```python
from build123d import *

# Parameters (mm, degrees)
SKETCH1_R           = 27.5
SKETCH1_R_2         = 2.5
BOSS_EXTRUDE1_DEPTH = 4
SKETCH2_R           = 11
CUT_EXTRUDE1_DEPTH  = 15
BOSS_EXTRUDE3_START = -4
SKETCH3_R           = 2.5
SKETCH3_R_2         = 1.875
BOSS_EXTRUDE3_DEPTH = 4


with BuildPart() as part:
    # Sketch1 → Boss-Extrude1 (new body)
    with BuildSketch(Plane(origin=(0, 0, 0), x_dir=(1, 0, 0), z_dir=(0, 1, 0))):
        with Locations(Location((0, 0, 0), (0, 0, 270))):
            Circle(SKETCH1_R)
        with Locations(Location((0, 20, 0), (0, 0, 270))):
            Circle(SKETCH1_R_2, mode=Mode.SUBTRACT)
        with Locations(Location((-20, 0, 0), (0, 0, 270))):
            Circle(SKETCH1_R_2, mode=Mode.SUBTRACT)
        with Locations(Location((20, 0, 0), (0, 0, 270))):
            Circle(SKETCH1_R_2, mode=Mode.SUBTRACT)
        with Locations(Location((0, -20, 0), (0, 0, 270))):
            Circle(SKETCH1_R_2, mode=Mode.SUBTRACT)
    extrude(amount=BOSS_EXTRUDE1_DEPTH)

    # Sketch2 → Cut-Extrude1 (cut)
    with BuildSketch(Plane(origin=(0, 4, 0), x_dir=(1, 0, 0), z_dir=(0, 1, 0))):
        with Locations(Location((0, 0, 0), (0, 0, 270))):
            Circle(SKETCH2_R)
    extrude(amount=-CUT_EXTRUDE1_DEPTH, mode=Mode.SUBTRACT)

    # Sketch3 → Boss-Extrude3 (add)
    # profile 1 of 4: a face of its own
    with BuildSketch(Plane(origin=(0, 4, 0), x_dir=(1, 0, 0), z_dir=(0, 1, 0)).offset(BOSS_EXTRUDE3_START)):
        with Locations((0, -20)):
            Circle(SKETCH3_R)
        with Locations(Location((0, -20, 0), (0, 0, 270))):
            Circle(SKETCH3_R_2, mode=Mode.SUBTRACT)
    # profile 2 of 4: a face of its own
    with BuildSketch(Plane(origin=(0, 4, 0), x_dir=(1, 0, 0), z_dir=(0, 1, 0)).offset(BOSS_EXTRUDE3_START)):
        with Locations((20, 0)):
            Circle(SKETCH3_R)
        with Locations(Location((20, 0, 0), (0, 0, 270))):
            Circle(SKETCH3_R_2, mode=Mode.SUBTRACT)
    # profile 3 of 4: a face of its own
    with BuildSketch(Plane(origin=(0, 4, 0), x_dir=(1, 0, 0), z_dir=(0, 1, 0)).offset(BOSS_EXTRUDE3_START)):
        with Locations((0, 20)):
            Circle(SKETCH3_R)
        with Locations(Location((0, 20, 0), (0, 0, 270))):
            Circle(SKETCH3_R_2, mode=Mode.SUBTRACT)
    # profile 4 of 4: a face of its own
    with BuildSketch(Plane(origin=(0, 4, 0), x_dir=(1, 0, 0), z_dir=(0, 1, 0)).offset(BOSS_EXTRUDE3_START)):
        with Locations((-20, 0)):
            Circle(SKETCH3_R)
        with Locations(Location((-20, 0, 0), (0, 0, 270))):
            Circle(SKETCH3_R_2, mode=Mode.SUBTRACT)
    extrude(amount=BOSS_EXTRUDE3_DEPTH)


solid = part.part
```
Geometry: final body of the model. Coordinates: model frame, mm. Round coordinates to 2 decimals unless told otherwise and drop trailing zeros. Write each loop counter-clockwise with the first axis right and the second up, starting at its lowest first coordinate (ties: lowest second). Pieces come first, ordered by that corner, then holes.
Item 1: Pin query (flat end, axial travel): P1, Ø1.5, axis at y = 3, z = 9.5, coming from the +X side. Return the tip coordinate at first contact, or that it passes through.
Item 2: Material intervals for L1, parallel to X at y = 1.4, z = 0 (3 decimals); L2, parallel to X at y = 3.4, z = 1; L3, parallel to Z at x = -21, y = 2.55, sorted ascending.
Item 3: Mould query, pull axis Z, two halves, no side actions, for faces 1 (the face through (-24.397, 1.972, 12.69)), 2 (the face through (0, 4, 12)), 3 (the face through (18.34, 1.97, 0.87)). Classes: +Z half, -Z half, draft (parallel to the pull), parting line (faces both ways), or undercut.
Item 4: Section query B-B (x = 0). Return loops of the section in (y, z) (3 decimals).
Item 5: Section query C-C (y = 2.2). Return loops of the section in (x, z) (3 decimals).
Item 6: Section query D-D (z = 9). Return loops of the section in (x, y), plus the area to 3 significant figures.
Item 7: Section query A-A (z = 0). Return loops of the section in (x, y) (3 decimals), plus the area to 3 significant figures.
Completed:
1. P1: stops at x = 26.07
2. L1: x = -27.5 to -21.875, -18.125 to -11, 11 to 18.125, 21.875 to 27.5
2. L2: x = -27.48 to -21.59, -18.41 to -10.95, 10.95 to 18.41, 21.59 to 27.48
2. L3: z = -17.76 to -1.59, 1.59 to 17.76
3. face 1: parting line
3. face 2: draft
3. face 3: undercut
4. outline: (0, -27.5) - (4, -27.5) - (4, -21.875) - (0, -21.875) - close; (0, -18.125) - (4, -18.125) - (4, -11) - (0, -11) - close; (0, 11) - (4, 11) - (4, 18.125) - (0, 18.125) - close; (0, 21.875) - (4, 21.875) - (4, 27.5) - (0, 27.5) - close
5. outline: circle Ø55 at (0, 0); hole circle Ø3.75 at (-20, 0); hole circle Ø22 at (0, 0); hole circle Ø3.75 at (0, -20); hole circle Ø3.75 at (0, 20); hole circle Ø3.75 at (20, 0)
6. outline: (-25.99, 0) - (-6.32, 0) - (-6.32, 4) - (-25.99, 4) - close; (6.32, 0) - (25.99, 0) - (25.99, 4) - (6.32, 4) - close
6. area: 157 mm2
7. outline: (-27.5, 0) - (-21.875, 0) - (-21.875, 4) - (-27.5, 4) - close; (-18.125, 0) - (-11, 0) - (-11, 4) - (-18.125, 4) - close; (11, 0) - (18.125, 0) - (18.125, 4) - (11, 4) - close; (21.875, 0) - (27.5, 0) - (27.5, 4) - (21.875, 4) - close
7. area: 102 mm2
